```python
from build123d import *

# Parameters (mm, degrees)
ESQUISSE1_W             = 250
ESQUISSE1_H             = 250
BOSS_EXTRU_1_DEPTH      = 96
CONG_1_R                = 32
ESQUISSE2_R             = 20
ESQUISSE2_R_2           = 5
ENL_V_MAT_EXTRU_1_DEPTH = 9.6


with BuildPart() as part:
    # Esquisse1 → Boss.-Extru.1 (new body)
    with BuildSketch(Plane.XY):
        Rectangle(ESQUISSE1_W, ESQUISSE1_H)
    extrude(amount=BOSS_EXTRU_1_DEPTH)

    # Congé1
    cong_1_edges = [part.edges().sort_by_distance(p)[0] for p in [
        (125, -125, 48),
        (-125, -125, 48),
        (-125, 125, 48),
        (125, 125, 48),
    ]]
    fillet(cong_1_edges, radius=CONG_1_R)

    # Esquisse2 → Enlèv. mat.-Extru.1 (cut)
    with BuildSketch(Plane.XY.offset(96)):
        with Locations((75, 75)):
            Circle(ESQUISSE2_R)
        with Locations((75, -75)):
            Circle(ESQUISSE2_R)
        with Locations((-62.5, 0)):
            Circle(ESQUISSE2_R_2)
    extrude(amount=-ENL_V_MAT_EXTRU_1_DEPTH, mode=Mode.SUBTRACT)


solid = part.part
```
Could you check a few things on this model? Use its own coordinates, in mm. A direction names the side the tool comes from. Coordinates: 2 decimals unless noted, no trailing zeros. Loops run counter-clockwise (first coordinate to the right, second up) from the corner with the lowest first, then second, coordinate; pieces in that order, holes last. Notation, with made-up numbers: M 53,28.5 L 111,28.5 A4 cw 111,34.5 Z; hole C -23,62 d9. An arc over 180 degrees is marked long. Put each result on its own line as item: value. Start each with the question number.
(1) For faces 1 (the face through (-1, 125, 47)), 2 (the face through (75, -75, 86.4)), which set-ups out of +Z, -Z, +X, -X, +Y, -Y let a thin tool reach every point of the face, with its end or its side?
(2) Thinking about a two-plate mould opening in X: for faces 3 (the face through (115.87, 115.38, 48.67)), 4 (the face through (-125, -1, 47)), 5 (the face through (-63, 0, 86.4)), which applies, pulls with the +X half, pulls with the -X half, needs draft (parallel to the pull), parting line crosses it, or undercut?
(3) Suppose I cut it at A-A on y = -75. Please give me the cut outline in (x, z), then the cut area to 3 significant figures.
(4) Suppose I cut it at B-B on y = 69. Please give me the cut outline in (x, z).
(5) I need wall thicknesses on line 1 (Y direction, x = 75, z = 90); line 2 (Y direction, x = -62.5, z = 93.5); line 3 (X direction, y = 93.5, z = 34). Which ranges of each line are inside material? Lowest first, please. Write a range as from..to.
(6) Will these pins go through, and if not, where does the flat tip stop? P1, Ø8, axis at x = -62.5, y = 0, coming from the +Z side; P2, Ø1.5, axis at y = -99, z = 15.5, coming from the -X side.
Solutions:
1. face 1: +Z, -Z, +X, -X, +Y
1. face 2: +Z
2. face 3: pulls with the +X half
2. face 4: pulls with the -X half
2. face 5: undercut
3. outline: M -125,0 L 125,0 L 125,96 L 95,96 L 95,86.4 L 55,86.4 L 55,96 L -125,96 Z
3. area: 23,600 mm2
4. outline: M -125,0 L 125,0 L 125,96 L 94.08,96 L 94.08,86.4 L 55.92,86.4 L 55.92,96 L -125,96 Z
5. line 1: y = -125..-95, -55..55, 95..125
5. line 2: y = -125..-5, 5..125
5. line 3: x = -125..125
6. P1: stops at z = 86.4
6. P2: stops at x = -124.57
